from build123d import *

# Parameters (mm, degrees)
SKETCH1_W           = 40
SKETCH1_H           = 4
SKETCH1_W_2         = 25
SKETCH1_H_2         = 17
BOSS_EXTRUDE1_DEPTH = 2
BOSS_EXTRUDE2_DEPTH = 0.5
SKETCH3_W           = 25
SKETCH3_H           = 2.5
BOSS_EXTRUDE3_DEPTH = 37
SKETCH4_R           = 8.5
CUT_EXTRUDE1_DEPTH  = 37
SKETCH6_W           = 12
SKETCH6_H           = 2.5
BOSS_EXTRUDE4_DEPTH = 30
SKETCH8_R           = 0.95
CUT_EXTRUDE2_DEPTH  = 30


with BuildPart() as part:
    # Sketch1 → Boss-Extrude1 (new body)
    with BuildSketch(Plane(origin=(0, 0, 0), x_dir=(1, 0, 0), z_dir=(0, 1, 0))):
        with Locations((-57.947101463, -109.729781289)):
            Rectangle(SKETCH1_W, SKETCH1_H)
        with Locations((-25.447101463, -109.729781289)):
            Rectangle(SKETCH1_W_2, SKETCH1_H_2)
        with Locations((7.052898537, -109.729781289)):
            Rectangle(SKETCH1_W, SKETCH1_H)
    extrude(amount=BOSS_EXTRUDE1_DEPTH)

    # Sketch2 → Boss-Extrude2 (add)
    with BuildSketch(Plane(origin=(0, 2, 0), x_dir=(1, 0, 0), z_dir=(0, 1, 0))):
        Polygon((-77.947101463, -108.397425258), (-62.457280687, -109.724520363), (-57.894492201, -109.335653269), (-76.638189664, -107.729781289), (-77.947101463, -107.729781289), align=None)
        Polygon((-76.638189664, -111.729781289), (-57.894492201, -110.115438654), (-62.457280687, -109.724520363), (-77.947101463, -111.044652036), (-77.947101463, -111.729781289), align=None)
        Polygon((-57.894492201, -110.115438654), (-39.051925459, -111.729781289), (-37.947101463, -111.729781289), (-37.947101463, -111.044652036), (-53.355645232, -109.724520363), align=None)
        Polygon((-62.457280687, -109.724520363), (-57.894492201, -110.115438654), (-53.355645232, -109.724520363), (-57.894492201, -109.335653269), align=None)
        Polygon((-57.894492201, -109.335653269), (-53.355645232, -109.724520363), (-37.947101463, -108.397425258), (-37.947101463, -107.729781289), (-39.051925459, -107.729781289), align=None)
        Polygon((-11.842277467, -111.729781289), (7.000289276, -110.115438654), (2.461442306, -109.724520363), (-12.947101463, -111.044652036), (-12.947101463, -111.729781289), align=None)
        Polygon((2.461442306, -109.724520363), (7.000289276, -109.335653269), (-11.842277467, -107.729781289), (-12.947101463, -107.729781289), (-12.947101463, -108.397425258), align=None)
        Polygon((7.000289276, -110.115438654), (11.563077761, -109.724520363), (7.000289276, -109.335653269), (2.461442306, -109.724520363), align=None)
        Polygon((27.052898537, -111.729781289), (27.052898537, -111.044652036), (11.563077761, -109.724520363), (7.000289276, -110.115438654), (25.743986738, -111.729781289), align=None)
        Polygon((7.000289276, -109.335653269), (11.563077761, -109.724520363), (27.052898537, -108.397425258), (27.052898537, -107.729781289), (25.743986738, -107.729781289), align=None)
    extrude(amount=BOSS_EXTRUDE2_DEPTH)

    # Sketch3 → Boss-Extrude3 (add)
    with BuildSketch(Plane(origin=(0, 2, 0), x_dir=(1, 0, 0), z_dir=(0, 1, 0))):
        with Locations((-25.447101463, -116.979781289)):
            Rectangle(SKETCH3_W, SKETCH3_H)
        with Locations((-25.447101463, -102.479781289)):
            Rectangle(SKETCH3_W, SKETCH3_H)
    extrude(amount=BOSS_EXTRUDE3_DEPTH)

    # Sketch4 → Cut-Extrude1 (cut)
    with BuildSketch(Plane.XY.offset(118.229781289)):
        with Locations(Location((-26.102234561, 29, 0), (0, 0, 180))):
            Circle(SKETCH4_R)
    extrude(amount=-CUT_EXTRUDE1_DEPTH, mode=Mode.SUBTRACT)

    # Sketch6 → Boss-Extrude4 (add)
    with BuildSketch(Plane(origin=(0, 39, 0), x_dir=(1, 0, 0), z_dir=(0, 1, 0))):
        with Locations((-25.447101463, -116.979781289)):
            Rectangle(SKETCH6_W, SKETCH6_H)
        with Locations((-25.447101463, -102.479781289)):
            Rectangle(SKETCH6_W, SKETCH6_H)
    extrude(amount=BOSS_EXTRUDE4_DEPTH)

    # Sketch8 → Cut-Extrude2 (cut)
    with BuildSketch(Plane.XY.offset(118.229781289)):
        with Locations(Location((-25.447101463, 66.872747416, 0), (0, 0, 180))):
            Circle(SKETCH8_R)
        with Locations(Location((-25.447101463, 61.774545812, 0), (0, 0, 180))):
            Circle(SKETCH8_R)
    extrude(amount=-CUT_EXTRUDE2_DEPTH, mode=Mode.SUBTRACT)


solid = part.part
Part model, mm, in its own coordinate system. A direction names the side the tool comes from. Give positions to 0.01 mm unless a question says otherwise; leave off trailing zeros. Write each loop counter-clockwise with the first axis right and the second up, starting at its lowest first coordinate (ties: lowest second). Pieces come first, ordered by that corner, then holes.
1) Which spindle directions (+Z, -Z, +X, -X, +Y, -Y) get a long thin tool onto all of the face, cutting with end or side? Do faces 5 (the face through (-31.447, 54, 102)), 6 (the face through (21, 2, 110)), 7 (the face through (-37.947, 15, 103)), 8 (the face through (-37.947, 19, 116)), 9 (the face through (-16, 39, 117)). Say none if no direction does.
Resolved:
face 5: +Z, -Z, -X, +Y
face 6: +X, +Y
face 7: -Z, -X, +Y, -Y
face 8: +Z, -X, +Y, -Y
face 9: +Z, -Z, +X, +Y
2) Two-plate mould, pull along Z, no slides. Class faces 1 (the face through (-17, 28, 103.73)), 2 (the face through (-72, 2, 110)), 3 (the face through (-17, 26, 101.23)), 4 (the face through (-24.26, 37.3, 102.5)): released by +Z, released by -Z, zero draft, split by the parting line, or undercut.
Resolved:
face 1: undercut
face 2: undercut
face 3: released by -Z
face 4: zero draft
3) Pin check, flat tips, straight feed: pin 1 (0.5 mm diameter, centred on x = 5.5, z = 111.5, fed in from +Y); pin 2 (10 mm diameter, centred on y = 26, z = 106.5, fed in from -X); pin 3 (0.8 mm diameter, centred on x = -64.5, z = 110.5, fed in from +Y). Stop position of each tip, or through.
Resolved:
pin 1: stops at y = 2
pin 2: stops at x = -37.95
pin 3: stops at y = 2.5
4) Probe L1, parallel to X at y = 29, z = 117.2; L2, parallel to Z at x = -20, y = 5; L3, parallel to X at y = 6, z = 117.75. List the from-to ranges inside material, lowest first.
Resolved:
L1: x = -37.95 to -34.6, -17.6 to -12.95
L2: z = 101.23 to 103.73, 115.73 to 118.23
L3: x = -37.95 to -12.95
5) Cut at C-C on x = -15. Write the cut outline in (y, z).
Resolved:
outline: (0, 101.23) - (39, 101.23) - (39, 103.73) - (2, 103.73) - (2, 115.73) - (39, 115.73) - (39, 118.23) - (0, 118.23) - close
6) Cut at D-D on z = 112.75. Write the cut outline in (x, y), then the cut area to 3 significant figures.
Resolved:
outline: (-37.95, 0) - (-12.95, 0) - (-12.95, 2) - (-37.95, 2) - close
area: 50.0 mm2
7) Cut at A-A on y = 52.5. Write the cut outline in (x, z), then the cut area to 3 significant figures.
Resolved:
outline: (-31.45, 101.23) - (-19.45, 101.23) - (-19.45, 103.73) - (-31.45, 103.73) - close; (-31.45, 115.73) - (-19.45, 115.73) - (-19.45, 118.23) - (-31.45, 118.23) - close
area: 60.0 mm2
8) Cut at B-B on y = 29. Write the cut outline in (x, z).
Resolved:
outline: (-37.95, 101.23) - (-34.6, 101.23) - (-34.6, 103.73) - (-37.95, 103.73) - close; (-37.95, 115.73) - (-34.6, 115.73) - (-34.6, 118.23) - (-37.95, 118.23) - close; (-17.6, 101.23) - (-12.95, 101.23) - (-12.95, 103.73) - (-17.6, 103.73) - close; (-17.6, 115.73) - (-12.95, 115.73) - (-12.95, 118.23) - (-17.6, 118.23) - close
